```python
from build123d import *


with BuildPart() as f1:
    # F0 (on Front) → F1 (revolve)
    with BuildSketch(Plane.XZ):
        with BuildLine():
            ThreePointArc((15.875, -11.2468861043), (19.5966413277, -6.152735897), (20.9912098944, 0))
            Line((20.9912098944, 0), (160.02, 0))
            Line((160.02, 0), (157.48, 6.35))
            Line((157.48, 6.35), (19.05, 6.35))
            add(Edge.make_bspline(
                [(19.05, 6.35), (17.2943395607, -5.2739201542), (10.3896663187, -7.9876436539), (9.4300154597, -16.612906009), (9.525, -23.8922853023)],
                knots=[0, 0, 0, 0, 0.5270987441, 1, 1, 1, 1], degree=3))
            Line((9.525, -23.8922853023), (9.525, -40.0551594794))
            add(Edge.make_bspline(
                [(15.875, -50.8), (14.4695304334, -45.8264946938), (9.4677070156, -44.9470542371), (9.525, -40.0551594794)],
                knots=[0, 0, 0, 0, 12.4809493955, 12.4809493955, 12.4809493955, 12.4809493955], degree=3))
            Line((15.875, -50.8), (15.875, -11.2468861043))
        make_face()
    revolve(axis=Axis((0, 0, 2.4035767974), (0, 0, -1)))


solid = f1.part
```
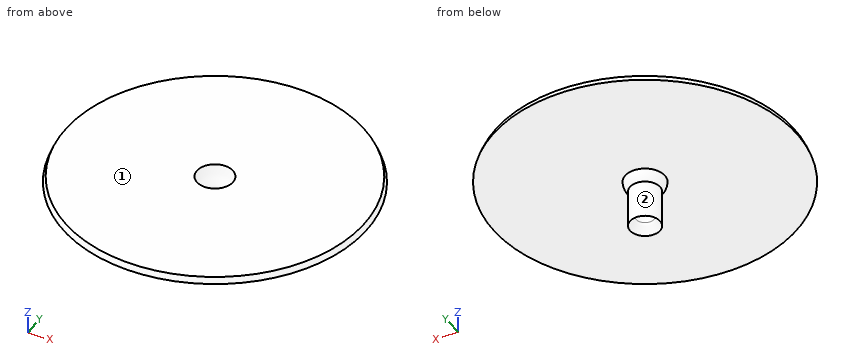
For this review, take the finished solid that the model builds, in its own axes (mm). Face numbers are marked on the shaded views. A direction names the side the tool comes from. Coordinates: 2 decimals unless noted, no trailing zeros. Write each loop counter-clockwise with the first axis right and the second up, starting at its lowest first coordinate (ties: lowest second). Pieces come first, ordered by that corner, then holes. Notation, with made-up numbers: (-11, 8.5) - (32, 8.5) arc R21 ccw to (32, 30.5) - close; hole circle Ø4 at (26, 73). An arc over 180 degrees is marked (long way). Answer in a Markdown table with one row per item. Add a question column.
Q1. Tool access review of the marked faces 1 and 2: name each direction out of +Z, -Z, +X, -X, +Y, -Y from which nothing blocks a thin tool from reaching the whole face with its end or side.
Q2. We need section A-A, the plane z = -28.5. State the section outline as (x, y) points (3 decimals), and give its area (3 significant figures).
Q3. For P1, Ø4, axis at x = 19, y = -6, coming from the -Z side; P2, Ø22, axis at x = 0, y = 0, coming from the -Z side; P3, Ø12, axis at y = -20, z = -29.5, coming from the +X side, all flat-tipped, find the tip position at first contact; note any pin that passes through.
Q4. For probe 1 along X at (y, z) = (0, -27) (3 decimals); probe 2 along Z at (x, y) = (40.5, 107.5), list the stretches that pass through material, from the lowest coordinate up.
Answer list:
| question | item | result |
|---|---|---|
| 1 | face 1 | +Z, +X, -X, +Y, -Y |
| 1 | face 2 | -Z |
| 2 | outline | circle Ø31.75 at (0, 0); hole circle Ø19.05 at (0, 0) |
| 2 | area | 507 mm2 |
| 3 | P1 | stops at z = -8.99 |
| 3 | P2 | stops at z = -44.12 |
| 3 | P3 | stops at x = 7.48 |
| 4 | probe 1 | x = -15.875 to -9.525, 9.525 to 15.875 |
| 4 | probe 2 | z = 0 to 6.35 |
